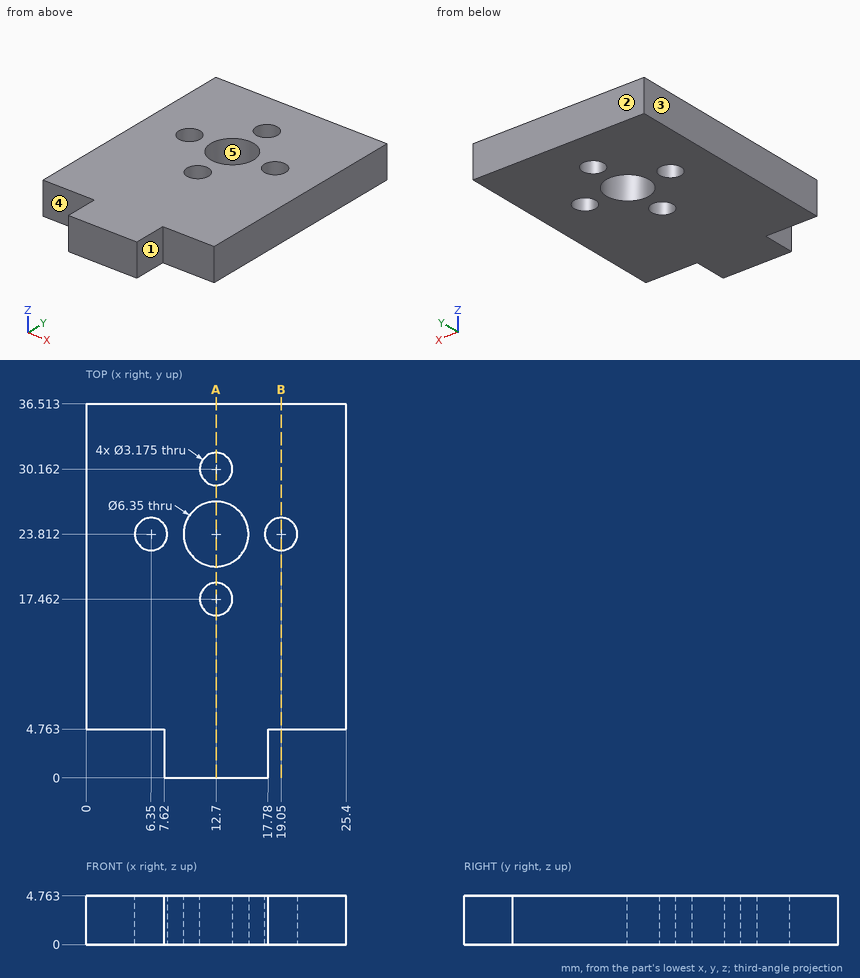
Design review of the part shown in the three views and the two pictorial views. Dimensions are in mm from the part's minimum x, y and z. A direction names the side the tool comes from. Give positions to 0.01 mm unless a question says otherwise; leave off trailing zeros. Loops run counter-clockwise (first coordinate to the right, second up) from the corner with the lowest first, then second, coordinate; pieces in that order, holes last. Notation, with made-up numbers: (9, -30.5) - (60, -30.5) arc R17 ccw to (60, -10.5) - close; hole circle Ø4 at (80.25, 27.25). An arc over 180 degrees is marked (long way). Answer as a JSON object with one key per item and string values.
Q1. Add section A-A on x = 12.7. Count the separate pieces of the cut face and the enclosed holes in it, plus the area to 3 significant figures.
Worked out:
{"separate pieces": "4", "enclosed holes": "0", "area": "113 mm^2"}
Q2. Insertion check: pin 1 (4 mm diameter, centred on x = 7.5, y = 20.5, fed in from -Z); pin 2 (2.5 mm diameter, centred on x = 3.5, z = 3, fed in from -Y); pin 3 (1.4 mm diameter, centred on y = 2.5, z = 2.5, fed in from +X). Each pin has a flat end and moves straight along its axis. Give the tip position at first contact, or say it passes through.
Worked out:
{"pin 1": "stops at z = 0", "pin 2": "stops at y = 4.76", "pin 3": "stops at x = 17.78"}
Q3. Mouldability with a two-part tool opening along Y and no side actions: class the marked faces 3, 4 and 5 as +Y half, -Y half, draft (parallel to the pull), parting line (faces both ways), or undercut.
Worked out:
{"face 3": "draft", "face 4": "-Y half", "face 5": "undercut"}
Q4. Add section B-B on x = 19.05. State the section outline as (y, z) points (1 decimal).
Worked out:
{"outline": "(4.8, 0) - (22.2, 0) - (22.2, 4.8) - (4.8, 4.8) - close; (25.4, 0) - (36.5, 0) - (36.5, 4.8) - (25.4, 4.8) - close"}
Q5. To check wall thickness, follow line 1 along X through (y, z) = (23.5, 2.55); line 2 along X through (y, z) = (30, 4.1); line 3 along X through (y, z) = (25, 2.5) (1 decimal). State the ranges of each line that lie inside material, in increasing order.
Worked out:
{"line 1": "x = 0 to 4.79, 7.91 to 9.54, 15.86 to 17.49, 20.61 to 25.4", "line 2": "x = 0 to 11.12, 14.28 to 25.4", "line 3": "x = 0 to 5.3, 7.4 to 9.8, 15.6 to 18, 20.1 to 25.4"}
Q6. For the marked faces 1 and 2, list the 3-axis set-ups (+Z, -Z, +X, -X, +Y, -Y) from which the entire face can be reached by the end or side of a thin tool; tool diameter is ignored.
Worked out:
{"face 1": "+Z, -Z, +X, -Y", "face 2": "+Z, -Z, +X, -X, +Y"}
